The model under review builds one solid part; all positions refer to its coordinate system, in mm. Face numbers are marked on the shaded views. Give positions to 0.01 mm unless a question says otherwise; leave off trailing zeros. Write each loop counter-clockwise with the first axis right and the second up, starting at its lowest first coordinate (ties: lowest second). Pieces come first, ordered by that corner, then holes.
from build123d import *

# Parameters (mm, degrees)
F0_W     = 67.1
F0_H     = 138.3
F1_DEPTH = 3.55
F2_R     = 5.08
F3_T     = -2.54
F4_W     = 24.637904
F4_H     = 11.145718
F5_DEPTH = 12.5
F6_W     = 14.344266
F6_H     = 7.1
F7_DEPTH = 3.5
F8_W     = 4.111376
F8_H     = 35.32717
F9_DEPTH = 12.5


with BuildPart() as f1:
    # F0 (on Front) → F1 (new body, symmetric)
    with BuildSketch(Plane.XZ):
        Rectangle(F0_W, F0_H)
    extrude(amount=F1_DEPTH, both=True)

    # F2
    f2_edges = [f1.edges().sort_by_distance(p)[0] for p in [
        (-33.55, 0, 69.15),
        (33.55, 0, 69.15),
        (33.55, 0, -69.15),
        (-33.55, 0, -69.15),
    ]]
    fillet(f2_edges, radius=F2_R)

    # F3
    f3_openings = [f1.faces().sort_by_distance(p)[0] for p in [
        (0, -3.55, 0),
    ]]
    offset(amount=F3_T, openings=f3_openings)

    # F4 (on face) → F5 (cut, symmetric)
    with BuildSketch(Plane(origin=(0, 3.55, 0), x_dir=(-1, 0, 0), z_dir=(0, 1, 0))):
        with Locations((-19.333094, 60.415514)):
            Rectangle(F4_W, F4_H)
    extrude(amount=F5_DEPTH, both=True, mode=Mode.SUBTRACT)

    # F6 (on face) → F7 (cut, symmetric)
    with BuildSketch(Plane(origin=(0, 0, -69.15), x_dir=(1, 0, 0), z_dir=(0, 0, -1))):
        Rectangle(F6_W, F6_H)
    extrude(amount=F7_DEPTH, both=True, mode=Mode.SUBTRACT)

    # F8 (on face) → F9 (cut, symmetric)
    with BuildSketch(Plane(origin=(-33.55, 0, 0), x_dir=(0, -1, 0), z_dir=(-1, 0, 0))):
        with Locations((0, 35.298977)):
            Rectangle(F8_W, F8_H)
    extrude(amount=F9_DEPTH, both=True, mode=Mode.SUBTRACT)


solid = f1.part
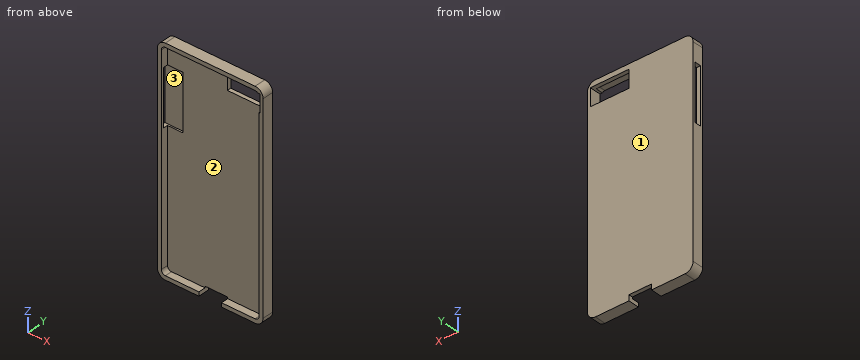
1) Consider section D-D, the plane x = -24. Give the boundary of the cut face in (y, z).
2) To check wall thickness, follow probe 1 along Z at (x, y) = (17.5, -0.75); probe 2 along X at (y, z) = (-1.25, 10); probe 3 along Z at (x, y) = (17, 3). State the ranges of each line that lie inside material, in increasing order.
3) Consider section C-C, the plane y = -0.25. Give the boundary of the cut face in (x, z).
4) Consider section A-A, the plane x = 16.5. Give the boundary of the cut face in (y, z).
5) The part is to be moulded in two halves that separate along Z. For the marked faces 1, 2 and 3, say which applies: +Z half, -Z half, draft (parallel to the pull), parting line (faces both ways), or undercut.
6) Consider section B-B, the plane z = 61. Give the boundary of the cut face in (x, y), then the cut area to 3 significant figures.
7) Insertion check: pin 1 (0.8 mm diameter, centred on x = 2, y = 1.5, fed in from -Z); pin 2 (4 mm diameter, centred on y = 0.5, z = -67, fed in from -X); pin 3 (4 mm diameter, centred on y = 0, z = -68.5, fed in from +X). Each pin has a flat end and moves straight along its axis. Give the tip position at first contact, or say it passes through.
Answer block:
1. outline: (-3.55, -69.15) - (3.55, -69.15) - (3.55, 69.15) - (-3.55, 69.15) - (-3.55, 66.61) - (1.01, 66.61) - (1.01, 52.96) - (2.06, 52.96) - (2.06, 17.64) - (1.01, 17.64) - (1.01, -66.61) - (-3.55, -66.61) - close
2. probe 1: z = -69.15 to -66.61, 66.61 to 69.15
2. probe 2: x = -33.55 to -31.01, 31.01 to 33.55
2. probe 3: z = -69.15 to 54.84, 65.99 to 69.15
3. outline: (-33.55, -64.07) arc R5.08 ccw to (-28.47, -69.15) - (-7.17, -69.15) - (-7.17, -66.61) - (-28.47, -66.61) arc R2.54 cw to (-31.01, -64.07) - (-31.01, 17.64) - (-33.55, 17.64) - close; (-33.55, 52.96) - (-31.01, 52.96) - (-31.01, 64.07) arc R2.54 cw to (-28.47, 66.61) - (28.47, 66.61) arc R2.54 cw to (30.13, 65.99) - (31.65, 65.99) - (31.65, 54.84) - (31.01, 54.84) - (31.01, -64.07) arc R2.54 cw to (28.47, -66.61) - (7.17, -66.61) - (7.17, -69.15) - (28.47, -69.15) arc R5.08 ccw to (33.55, -64.07) - (33.55, 64.07) arc R5.08 ccw to (28.47, 69.15) - (-28.47, 69.15) arc R5.08 ccw to (-33.55, 64.07) - close
4. outline: (-3.55, -69.15) - (3.55, -69.15) - (3.55, 54.84) - (1.01, 54.84) - (1.01, -66.61) - (-3.55, -66.61) - close; (-3.55, 66.61) - (1.01, 66.61) - (1.01, 65.99) - (3.55, 65.99) - (3.55, 69.15) - (-3.55, 69.15) - close
5. face 1: draft
5. face 2: undercut
5. face 3: undercut
6. outline: (-33.55, -3.55) - (-31.01, -3.55) - (-31.01, 1.01) - (7.01, 1.01) - (7.01, 3.55) - (-33.55, 3.55) - close; (31.65, -3.55) - (33.55, -3.55) - (33.55, 3.55) - (31.65, 3.55) - close
6. area: 128 mm2
7. pin 1: stops at z = -65.65
7. pin 2: stops at x = -33.46
7. pin 3: stops at x = 32.93
